Read the model definition and answer for the solid it produces. Units are mm, in the model's axes. A direction names the side the tool comes from. Give positions to 0.01 mm unless a question says otherwise; leave off trailing zeros. Write each loop counter-clockwise with the first axis right and the second up, starting at its lowest first coordinate (ties: lowest second). Pieces come first, ordered by that corner, then holes. Notation, with made-up numbers: (-33.5, 85) -> (-6.5, 85) arc R28 ccw to (-6.5, 113) -> close; hole circle Ø2 at (-18.5, 31.5). An arc over 180 degrees is marked (long way). Put each result on its own line as item: value. Start each with the question number.
from build123d import *

# Parameters (mm, degrees)
SKETCH1_W           = 38.1
SKETCH1_H           = 2.286
BOSS_EXTRUDE1_DEPTH = 4.064
SKETCH3_W           = 38.1
SKETCH3_H           = 2.54
BOSS_EXTRUDE3_DEPTH = 7.112
SKETCH4_W           = 0.762
SKETCH4_H           = 1.016
CUT_EXTRUDE1_DEPTH  = 30.734


with BuildPart() as part:
    # Sketch1 → Boss-Extrude1 (new body)
    with BuildSketch(Plane(origin=(0, 0, 0), x_dir=(1, 0, 0), z_dir=(0, 1, 0))):
        with Locations((-8.736060606, 1.550939394)):
            Rectangle(SKETCH1_W, SKETCH1_H)
    extrude(amount=BOSS_EXTRUDE1_DEPTH)

    # Sketch3 → Boss-Extrude3 (add)
    with BuildSketch(Plane(origin=(0, 0, -2.693939394), x_dir=(-1, 0, 0), z_dir=(0, 0, -1))):
        with Locations((8.736060606, 0.254)):
            Rectangle(SKETCH3_W, SKETCH3_H)
    extrude(amount=BOSS_EXTRUDE3_DEPTH)

    # Sketch4 → Cut-Extrude1 (cut)
    with BuildSketch(Plane.ZY.offset(27.786060606)):
        with Locations((-3.074939394, -0.508)):
            Rectangle(SKETCH4_W, SKETCH4_H)
    extrude(amount=-CUT_EXTRUDE1_DEPTH, mode=Mode.SUBTRACT)


solid = part.part
1) A cutting plane is placed at A-A on x = 0.5. Give the vertices of the cut face in (y, z).
2) Each of these flat-tipped pins is pushed along its axis until it touches: pin 1 Ø1.3 at (x, y) = (-2, 2.5) entering from -Z; pin 2 Ø0.5 at (x, y) = (-16, -0.5) entering from +Z; pin 3 Ø2 at (x, z) = (5, -4) entering from +Y. Where does it stop, or does it pass through?
3) A cutting plane is placed at C-C on z = -1.5. Give the vertices of the cut face in (x, y), and give its area (3 significant figures).
4) A cutting plane is placed at B-B on y = 3.3. Give the vertices of the cut face in (x, z), and give its area (3 significant figures).
5) For faces 1 (the face through (6.7, -0.5, -2.694)), 2 (the face through (-12.6, -0.5, -3.456)), 3 (the face through (-9, 3, -2.694)), determine the directions among +Z, -Z, +X, -X, +Y, -Y from which every point of the face is accessible in a straight line to the end or side of a thin tool.
6) Straight lines are drawn through the part: line 1 (Y direction, x = -6, z = -2); line 2 (Z direction, x = -18.5, y = 3.8); line 3 (Y direction, x = -15, z = -8.25). For each, find the intervals that lie inside material, in ascending order. Write a range as [from, to].
Results found:
1. outline: (-1.02, -9.81) -> (1.52, -9.81) -> (1.52, -2.69) -> (4.06, -2.69) -> (4.06, -0.41) -> (0, -0.41) -> (0, -3.46) -> (-1.02, -3.46) -> close
2. pin 1: stops at z = -2.69
2. pin 2: stops at z = -3.46
2. pin 3: stops at y = 1.52
3. outline: (-27.79, 0) -> (10.31, 0) -> (10.31, 4.06) -> (-27.79, 4.06) -> close
3. area: 155 mm²
4. outline: (-27.79, -2.69) -> (10.31, -2.69) -> (10.31, -0.41) -> (-27.79, -0.41) -> close
4. area: 87.1 mm²
5. face 1: +Z, +X, -X, -Y
5. face 2: +Z, -X, -Y
5. face 3: -Z, +X, -X, +Y
6. line 1: y = [0, 4.06]
6. line 2: z = [-2.69, -0.41]
6. line 3: y = [-1.02, 1.52]
